Geometry: final body of the model. Coordinates: model frame, mm. Give positions to 0.01 mm unless a question says otherwise; leave off trailing zeros. Loops run counter-clockwise (first coordinate to the right, second up) from the corner with the lowest first, then second, coordinate; pieces in that order, holes last. Notation, with made-up numbers: (40.25, 64.5) -> (94.25, 64.5) arc R20 cw to (94.25, 73.5) -> close; hole circle Ø5 at (41, 4). An arc over 180 degrees is marked (long way). Answer in a Markdown table with one row per item. Add a question column.
from build123d import *

# Parameters (mm, degrees)
SKETCH006_W             = 94
SKETCH006_H             = 30
PAD002_DEPTH            = 3
SKETCH008_R             = 8
HOLE002_DEPTH           = 25
SKETCH007_R             = 1.35
HOLE003_DEPTH           = 25
FILLET001_R             = 1
BODY001_PLACEMENT_ANGLE = 180


with BuildPart() as part:
    # Sketch006 → Pad002 (new body)
    with BuildSketch(Plane(origin=(0, 0, -13), x_dir=(1, 0, 0), z_dir=(0, 0, -1))):
        with Locations((107, 0)):
            Rectangle(SKETCH006_W, SKETCH006_H)
    extrude(amount=-PAD002_DEPTH)

    # Sketch008 (on Face6 of Pad002) → Hole002 (cut)
    with BuildSketch(Plane.XY.offset(-10)):
        with Locations((76.5, 0)):
            Circle(SKETCH008_R)
        with Locations((137.5, 0)):
            Circle(SKETCH008_R)
    extrude(amount=-HOLE002_DEPTH, mode=Mode.SUBTRACT)

    # Sketch007 (on Face5 of Pad002) → Hole003 (cut)
    with BuildSketch(Plane(origin=(0, 0, -13), x_dir=(1, 0, 0), z_dir=(0, 0, -1))):
        with Locations((64, -11)):
            Circle(SKETCH007_R)
        with Locations((64, 11)):
            Circle(SKETCH007_R)
        with Locations((150, 11)):
            Circle(SKETCH007_R)
        with Locations((150, -11)):
            Circle(SKETCH007_R)
    extrude(amount=-HOLE003_DEPTH, mode=Mode.SUBTRACT)

    # Fillet001
    fillet001_edges = [part.edges().sort_by_distance(p)[0] for p in [
        (154, -15, -11.5),
        (154, 15, -11.5),
        (60, 15, -11.5),
        (60, -15, -11.5),
    ]]
    fillet(fillet001_edges, radius=FILLET001_R)


with BuildPart() as part_1:
    # Body001 placement: moved
    add(part.part.moved(Location((0, 0, -13))).rotate(Axis((0, 0, -13), (0, 1, 0)), BODY001_PLACEMENT_ANGLE))


solid = part_1.part
(1) Cut plane C-C on x = -137.5. Return the cut outline in (y, z), then the cut area to 3 significant figures.
(2) Pin query (flat end, axial travel): pin 1 Ø2 at (x, y) = (-64, 11) entering from +Z. Return the tip coordinate at first contact, or that it passes through.
(3) Draft query along Y for faces 1 (the flat face through (-154, 0, -1)), 2 (the flat face through (-106, -15, -1)), 3 (the cylindrical face through (-151.288, 10.594, -1.479)). Return one class per face: +Y half, -Y half, draft (parallel to the pull), parting line (faces both ways), or undercut.
(4) Material intervals for line 1 along Y through (x, z) = (-150, -1.85); line 2 along X through (y, z) = (-11, -0.8); line 3 along Y through (x, z) = (-77, -1.7), sorted ascending. Write a range as from..to.
(5) Cut plane A-A on y = 0. Return the cut outline in (x, z).
(6) Cut plane D-D on z = -2.5. Return the cut outline in (x, y), then the cut area to 3 significant figures.
(7) Cut plane B-B on x = -150. Return the cut outline in (y, z), then the cut area to 3 significant figures.
Answer list:
| question | item | result |
|---|---|---|
| 1 | outline | (-15, -3) -> (-8, -3) -> (-8, 0) -> (-15, 0) -> close; (8, -3) -> (15, -3) -> (15, 0) -> (8, 0) -> close |
| 1 | area | 42.0 mm² |
| 2 | pin 1 | passes through |
| 3 | face 1 | draft |
| 3 | face 2 | -Y half |
| 3 | face 3 | undercut |
| 4 | line 1 | y = -15..-12.35, -9.65..9.65, 12.35..15 |
| 4 | line 2 | x = -154..-151.35, -148.65..-65.35, -62.65..-60 |
| 4 | line 3 | y = -15..-7.98, 7.98..15 |
| 5 | outline | (-154, -3) -> (-145.5, -3) -> (-145.5, 0) -> (-154, 0) -> close; (-129.5, -3) -> (-84.5, -3) -> (-84.5, 0) -> (-129.5, 0) -> close; (-68.5, -3) -> (-60, -3) -> (-60, 0) -> (-68.5, 0) -> close |
| 6 | outline | (-154, -14) arc R1 ccw to (-153, -15) -> (-61, -15) arc R1 ccw to (-60, -14) -> (-60, 14) arc R1 ccw to (-61, 15) -> (-153, 15) arc R1 ccw to (-154, 14) -> close; hole circle Ø2.7 at (-150, -11); hole circle Ø2.7 at (-150, 11); hole circle Ø16 at (-137.5, 0); hole circle Ø16 at (-76.5, 0); hole circle Ø2.7 at (-64, -11); hole circle Ø2.7 at (-64, 11) |
| 6 | area | 2,390 mm² |
| 7 | outline | (-15, -3) -> (-12.35, -3) -> (-12.35, 0) -> (-15, 0) -> close; (-9.65, -3) -> (9.65, -3) -> (9.65, 0) -> (-9.65, 0) -> close; (12.35, -3) -> (15, -3) -> (15, 0) -> (12.35, 0) -> close |
| 7 | area | 73.8 mm² |
